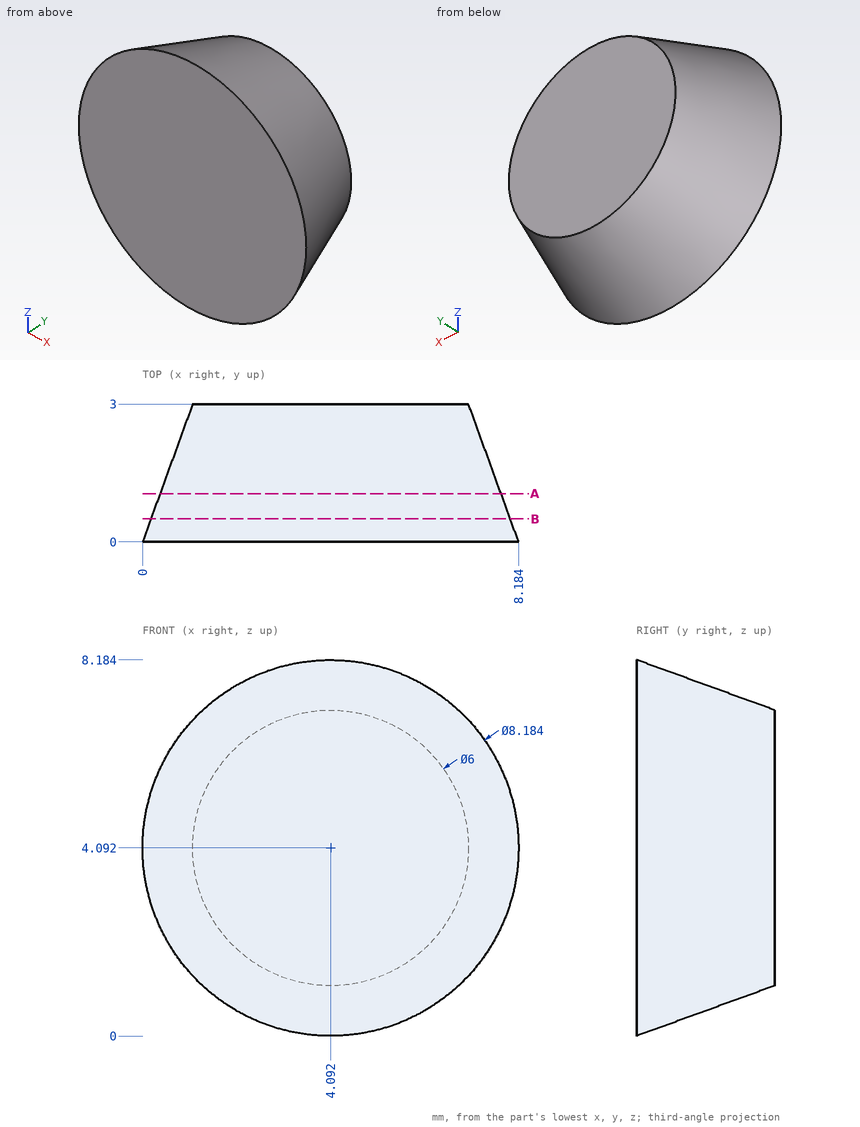
Design review of the part shown in the three views and the two pictorial views. Dimensions are in mm from the part's minimum x, y and z. Coordinates: 2 decimals unless noted, no trailing zeros. Order: outer loops, then holes, each group sorted by start corner. A loop starts at its lowest first (then second) coordinate and runs counter-clockwise, first axis right, second up.
1) Take a section at A-A, the plane y = 1.05. Give the boundary of the cut face in (x, z).
2) Take a section at B-B, the plane y = 0.5. Give the boundary of the cut face in (x, z).
3) Wall thickness on line 1 along X through (y, z) = (0.6, 5); line 2 along Z through (x, y) = (1, 2) (1 decimal); line 3 along Z through (x, y) = (6.5, 1.85) (1 decimal): over which ranges is each line inside the solid? List them lowest first.
Returned:
1. outline: circle Ø7.42 at (4.09, 4.09)
2. outline: circle Ø7.82 at (4.09, 4.09)
3. line 1: x = 0.33 to 7.86
3. line 2: z = 2.8 to 5.4
3. line 3: z = 1.7 to 6.5
